Autodesk Fusion 360 part; units mm, degrees
sketch "Sketch1" plane through (0, 0, 0) normal (0, 0, 1) x (1, 0, 0)
  line L0 (49, -21) -> (-49, -21)
  line L1 (-49, -21) -> (-49, 21)
  line L2 (-49, 21) -> (49, 21)
  line L3 (49, 21) -> (49, -21)
  line L4 (49, -21) -> (-49, 21) construction
  line L5 (-49, -21) -> (49, 21) construction
  dimension "d1" = 98
  dimension "d2" = 42
extrude "Extrude1" add sketch "Sketch1" along normal blind 20
sketch "Sketch2" plane through (0, -21, 0) normal (0, -1, 0) x (1, 0, 0)
  line L0 (-49, 0) -> (49, 0)
  line L1 (49, 0) -> (49, 20)
  line L2 (49, 20) -> (-49, 20)
  line L3 (-49, 20) -> (-49, 0)
  line L4 (-35, 0) -> (35, 0)
  line L5 (35, 0) -> (35, 6)
  line L6 (35, 6) -> (-35, 6)
  line L7 (-35, 6) -> (-35, 0)
  dimension "d5" = 6
  dimension "d6" = 14
  dimension "d7" = 14
extrude "Extrude2" cut sketch "Sketch2" against normal through all contours L0 L4 L5 L6 L7
sketch "Sketch3" plane through (0, 0, 20) normal (0, 0, 1) x (-1, 0, 0)
  line L0 (-49, -21) -> (49, -21)
  line L1 (49, -21) -> (49, 21)
  line L2 (49, 21) -> (-49, 21)
  line L3 (-49, 21) -> (-49, -21)
  line L4 (-7, 21) -> (7, 21)
  line L5 (7, 21) -> (7, -21)
  line L6 (7, -21) -> (-7, -21)
  line L7 (-7, -21) -> (-7, 21)
  line L8 (-7, 21) -> (7, -21) construction
  line L9 (7, 21) -> (-7, -21) construction
  dimension "d9" = 14
  dimension "d10" = 42
extrude "Extrude3" add sketch "Sketch3" along normal blind 42 contours L0 L2 L4 L5 L6 L7
fillet "Fillet1" radius 21 2 edges at (0, -21, 62) (0, 21, 62)
sketch "Sketch4" plane through (7, 0, 0) normal (1, 0, 0) x (0, 1, 0)
  arc A0 (21, 41) -> (-21, 41) centre (0, 41) ccw
  line L0 (-21, 41) -> (-21, 20)
  line L1 (-21, 20) -> (21, 20)
  line L2 (21, 20) -> (21, 41)
  circle A1 centre (0, 41) radius 10
  dimension "d15" = 20
extrude "Extrude4" cut sketch "Sketch4" against normal through all contours A1
sketch "Sketch5" plane through (0, 0, 20) normal (0, 0, 1) x (-1, 0, 0)
  line L0 (-7, -21) -> (-7, 21)
  line L1 (-7, 21) -> (-49, 21)
  line L2 (-49, 21) -> (-49, -21)
  line L3 (-49, -21) -> (-7, -21)
  circle A0 centre (-25, 0) radius 6
  dimension "d17" = 12
extrude "Extrude5" cut sketch "Sketch5" against normal through all contours A0
mirror "Mirror1" about plane through (0, 0, 0) normal (1, 0, 0) of "Extrude5"
fillet "Fillet2" radius 4 8 edges at (-49, 0, 20) (-7, -21, 30.5) (-7, 0, 62) (-7, 21, 30.5) (7, -21, 30.5) (7, 0, 62) (7, 21, 30.5) (49, 0, 20)
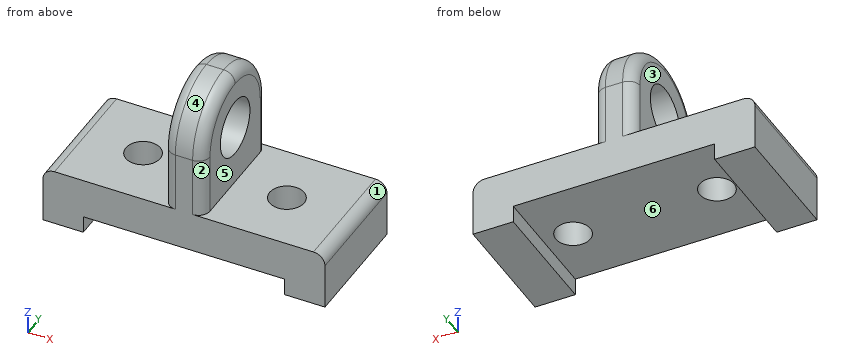
Part model, mm, in its own coordinate system. Face numbers are marked on the shaded views. A direction names the side the tool comes from. Round coordinates to 2 decimals unless told otherwise and drop trailing zeros. Loops run counter-clockwise (first coordinate to the right, second up) from the corner with the lowest first, then second, coordinate; pieces in that order, holes last.
Item 1: 3-axis set-ups, long thin cutter, end or side, ignore diameter. For the marked faces 1, 2 and 3: which of +Z, -Z, +X, -X, +Y, -Y reach the whole face in a straight line?
Item 2: Cut at B-B, the plane x = -25. Give the cut face in (y, z), then the cut area to 3 significant figures.
Item 3: Cut at C-C, the plane z = 4.5. Give the cut face in (x, y).
Item 4: Mould opens along X. For the marked faces 4, 5 and 6 say: +X half, -X half, draft (parallel to the pull), parting line (faces both ways), or undercut.
Item 5: Cut at A-A, the plane z = 33. Give the cut face in (x, y), then the cut area to 3 significant figures.
Item 6: Drill centre lines: line 1 (Y direction, x = -25, z = 15.75); line 2 (X direction, y = -5, z = 15.5); line 3 (X direction, y = 0, z = 17). Where is each one in solid material? Low to high.
Item 7: Cut at D-D, the plane y = 4. State how many separate pieces and enclosed holes the cut face has, then the cut area to 3 significant figures.
Item 8: Drop flat-ended pins along their axis: P1, Ø5, axis at x = -7, y = 4, coming from the -Z side; P2, Ø1.5, axis at x = 10, y = 4, coming from the +Z side; P3, Ø4, axis at y = -7, z = 38, coming from the -X side; P4, Ø1.5, axis at x = 4, y = -14.5, coming from the +Z side. Give the stop position or say it passes through.
A:
1. face 1: +Z, +X, +Y, -Y
1. face 2: +Z, +X, -Y
1. face 3: +Z, -X, +Y, -Y
2. outline: (-21, 6) - (-6, 6) - (-6, 20) - (-21, 20) - close; (6, 6) - (21, 6) - (21, 20) - (6, 20) - close
2. area: 420 mm2
3. outline: (-49, -21) - (-35, -21) - (-35, 21) - (-49, 21) - close; (35, -21) - (49, -21) - (49, 21) - (35, 21) - close
4. face 4: draft
4. face 5: +X half
4. face 6: undercut
5. outline: (-7, -17) arc R4 ccw to (-3, -21) - (3, -21) arc R4 ccw to (7, -17) - (7, -6) - (-7, -6) - close; (-7, 6) - (7, 6) - (7, 17) arc R4 ccw to (3, 21) - (-3, 21) arc R4 ccw to (-7, 17) - close
5. area: 406 mm2
6. line 1: y = -21 to -6, 6 to 21
6. line 2: x = -49 to -28.32, -21.68 to 21.68, 28.32 to 49
6. line 3: x = -48.87 to -31, -19 to 19, 31 to 48.87
7. separate pieces: 4
7. enclosed holes: 0
7. area: 1,600 mm2
8. P1: stops at z = 6
8. P2: stops at z = 20
8. P3: passes through
8. P4: stops at z = 56.74
